Could you check a few things on this model? Use its own coordinates, in mm. Round coordinates to 2 decimals unless told otherwise and drop trailing zeros. Order: outer loops, then holes, each group sorted by start corner. A loop starts at its lowest first (then second) coordinate and runs counter-clockwise, first axis right, second up. Notation, with made-up numbers: (-12.5, 25) - (24.5, 25) arc R11 cw to (24.5, 37) - close; hole circle Ø9 at (65.25, -18.75). An arc over 180 degrees is marked (long way). Return JSON: item names as keys, results as strings. Group by question number.
from build123d import *

# Parameters (mm, degrees)
SKETCH1_R               = 3
SKETCH1_R_2             = 2
BOSS_EXTRUDE1_DEPTH     = 6
SKETCH3_R               = 2.254
CUT_EXTRUDE1_DEPTH      = 0.254
CUT_EXTRUDE1_DRAFT      = -45
MIRROR1_COPY_1_SKETCH_R = 2.254
MIRROR1_COPY_1_DEPTH    = 0.254
MIRROR1_COPY_1_DRAFT    = -45


with BuildPart() as part:
    # Sketch1 → Boss-Extrude1 (new body)
    with BuildSketch(Plane(origin=(0, 0, 0), x_dir=(1, 0, 0), z_dir=(0, 1, 0))):
        with Locations(Location((0, 0, 0), (0, 0, 270))):
            Circle(SKETCH1_R)
        with Locations(Location((0, 0, 0), (0, 0, 270))):
            Circle(SKETCH1_R_2, mode=Mode.SUBTRACT)
    extrude(amount=BOSS_EXTRUDE1_DEPTH)


with BuildPart() as cut_extrude1_tool:
    # Sketch3 → Cut-Extrude1 (with draft: the straight prism first)
    with BuildSketch(Plane(origin=(0, 6, 0), x_dir=(1, 0, 0), z_dir=(0, 1, 0))):
        Circle(SKETCH3_R)
    extrude(amount=-CUT_EXTRUDE1_DEPTH)
    # Cut-Extrude1: the draft: its side faces are tilted about the plane it starts from
    cut_extrude1_sides = [cut_extrude1_tool.faces().sort_by_distance(p)[0] for p in [
        (-2.254, 5.873, 0),
    ]]
    draft(cut_extrude1_sides, Plane(origin=(0, 6, 0), x_dir=(1, 0, 0), z_dir=(0, 1, 0)), CUT_EXTRUDE1_DRAFT)


with BuildPart() as part_1:
    add(part.part)

    # Cut-Extrude1: cut by cut_extrude1_tool
    add(cut_extrude1_tool.part, mode=Mode.SUBTRACT)


with BuildPart() as mirror1_copy_1_tool:
    # Mirror1 copy 1 sketch → Mirror1 copy 1 (with draft: the straight prism first)
    with BuildSketch(Plane.XZ):
        Circle(MIRROR1_COPY_1_SKETCH_R)
    extrude(amount=-MIRROR1_COPY_1_DEPTH)
    # Mirror1 copy 1: the draft: its side faces are tilted about the plane it starts from
    mirror1_copy_1_sides = [mirror1_copy_1_tool.faces().sort_by_distance(p)[0] for p in [
        (-2.254, 0.127, 0),
    ]]
    draft(mirror1_copy_1_sides, Plane.XZ, MIRROR1_COPY_1_DRAFT)


with BuildPart() as part_2:
    add(part_1.part)

    # Mirror1 copy 1: cut by mirror1_copy_1_tool
    add(mirror1_copy_1_tool.part, mode=Mode.SUBTRACT)


solid = part_2.part
1) I want a section at C-C, the plane y = 5.6. List the corners of the cut face in (x, z) for me.
2) We'd pull the mould along X, two halves only. Please class faces 1 (the cylindrical face through (0.601, 2.962, 1.908)), 2 (the cylindrical face through (0.9, 2.96, 2.86)): +X half, -X half, draft (parallel to the pull), parting line (faces both ways), or undercut.
3) I want a section at B-B, the plane z = 0. List the corners of the cut face in (x, y) for me, plus the area to 3 significant figures.
4) I want a section at A-A, the plane x = 0. List the corners of the cut face in (y, z) for me, plus the area to 3 significant figures.
5) Will this pin go through, and if not, where does the flat tip stop? pin 1 (3 mm diameter, centred on y = 2.5, z = 2.5, fed in from -X).
6) I want a section at D-D, the plane z = 2.4. List the corners of the cut face in (x, y) for me.
7) If I drill on line 1 along X through (y, z) = (1.2, 0); line 2 along Z through (x, y) = (-0.7, 2); line 3 along Z through (x, y) = (-1.25, 4.6), over which ranges is the centre line in solid material (lowest first)? Write a range as from..to.
Outcome:
{
 "1": {"outline": "circle Ø6 at (0, 0); hole circle Ø4 at (0, 0)"},
 "2": {"face 1": "undercut", "face 2": "parting line"},
 "3": {"outline": "(-3, 0) - (-2.25, 0) - (-2, 0.25) - (-2, 5.75) - (-2.25, 6) - (-3, 6) - close; (2, 0.25) - (2.25, 0) - (3, 0) - (3, 6) - (2.25, 6) - (2, 5.75) - close", "area": "11.9 mm^2"},
 "4": {"outline": "(0, -3) - (6, -3) - (6, -2.25) - (5.75, -2) - (0.25, -2) - (0, -2.25) - close; (0, 2.25) - (0.25, 2) - (5.75, 2) - (6, 2.25) - (6, 3) - (0, 3) - close", "area": "11.9 mm^2"},
 "5": {"pin 1": "x = -2.83"},
 "6": {"outline": "(-1.8, 0) - (1.8, 0) - (1.8, 6) - (-1.8, 6) - close"},
 "7": {"line 1": "-3..-2, 2..3", "line 2": "-2.92..-1.87, 1.87..2.92", "line 3": "-2.73..-1.56, 1.56..2.73"}
}
